Build history of the part. All positions in model axes, mm. A direction names the side the tool comes from. Round coordinates to 2 decimals unless told otherwise and drop trailing zeros. Write each loop counter-clockwise with the first axis right and the second up, starting at its lowest first coordinate (ties: lowest second). Pieces come first, ordered by that corner, then holes. Notation, with made-up numbers: (41, 64) -> (52, 64) arc R8 ccw to (52, 69) -> close; hole circle Ø5 at (48.5, -34.75). An arc over 180 degrees is marked (long way). Answer in a Markdown table with one row per item.
```python
from build123d import *

# Parameters (mm, degrees)
F0_R     = 1.875
F1_DEPTH = 10
F2_R     = 1.15
F3_DEPTH = 25
F6_SIZE  = 0.5


with BuildPart() as f1:
    # F0 (on Top) → F1 (new body)
    with BuildSketch(Plane.XY):
        Circle(F0_R)
    extrude(amount=F1_DEPTH)

    # F2 (on face) → F3 (cut)
    with BuildSketch(Plane.XY.offset(10)):
        Circle(F2_R)
    extrude(amount=-F3_DEPTH, mode=Mode.SUBTRACT)

    # F4 (on Front) → F5 (revolve)
    with BuildSketch(Plane.XZ):
        Polygon((1.738653, 6), (1.783498, 4), (2.783498, 4), (2.783498, 6), align=None)
    revolve(axis=Axis((0, 0, 3.566666), (0, 0, 1)))

    # F6
    f6_edges = [f1.edges().sort_by_distance(p)[0] for p in [
        (-2.783498, 0, 4),
        (-2.783498, 0, 6),
    ]]
    chamfer(f6_edges, length=F6_SIZE)


solid = f1.part
```
Q1. Wall check: line 1 (Y direction, x = 0, z = 6.25) (3 decimals); line 2 (Y direction, x = -0.6, z = 2.5); line 3 (X direction, y = -0.2, z = 6.75). Give the ranges that are in metal, low to high. Write a range as [from, to].
A:
| item | result |
|---|---|
| line 1 | [-1.875, -1.15], [1.15, 1.875] |
| line 2 | [-1.78, -0.98], [0.98, 1.78] |
| line 3 | [-1.86, -1.13], [1.13, 1.86] |
Q2. Two-plate mould, pull along X, no slides. Class faces 3 (the cylindrical face through (-1.873, 0.082, 7.972)), 4 (the flat face through (1, 1, 0)), 5 (the cylindrical face through (-0.91, -0.7, 5.07)): released by +X, released by -X, zero draft, split by the parting line, or undercut.
A:
| item | result |
|---|---|
| face 3 | split by the parting line |
| face 4 | zero draft |
| face 5 | undercut |
Q3. Drop flat-ended pins along their axis: P1, Ø1.5, axis at x = 0, z = 8.5, coming from the -Y side (3 decimals); P2, Ø1, axis at x = 2, z = 8.5, coming from the +Y side (3 decimals). Give the stop position or say it passes through.
A:
| item | result |
|---|---|
| P1 | y = -1.875 |
| P2 | y = 1.125 |
Q4. Which spindle directions (+Z, -Z, +X, -X, +Y, -Y) get a long thin tool onto all of the face, cutting with end or side? Do faces 1 (the flat face through (1, 1, 10)), 2 (the cylindrical face through (-1.873, 0.082, 1.972)). Say none if no direction does.
A:
| item | result |
|---|---|
| face 1 | +Z, +X, -X, +Y, -Y |
| face 2 | -Z |
Q5. Saw through at C-C on z = 6.75. Write the cut outline in (x, y) (3 decimals), plus the area to 3 significant figures.
A:
| item | result |
|---|---|
| outline | circle Ø3.75 at (0, 0); hole circle Ø2.3 at (0, 0) |
| area | 6.89 mm² |
